```python
from build123d import *

# Parameters (mm, degrees)
F0_W     = 449.58
F0_H     = 176.784
F1_DEPTH = 70.866
F2_R     = 38.835317
F2_R_2   = 41.172166
F3_DEPTH = 25.4


with BuildPart() as f1:
    # F0 (on Top) → F1 (new body)
    with BuildSketch(Plane.XY):
        with Locations((-0.463787, -9.675345)):
            Rectangle(F0_W, F0_H)
    extrude(amount=F1_DEPTH)

    # F2 (on Front) → F3 (join)
    with BuildSketch(Plane.XZ):
        with Locations((-143.220037, 0)):
            Circle(F2_R)
        with Locations((175.135151, 0)):
            Circle(F2_R_2)
    extrude(amount=F3_DEPTH)


solid = f1.part
```
Input: part model. Units: mm. Frame: model coordinates. A direction names the side the tool comes from. Coordinates: 2 decimals unless noted, no trailing zeros. Loops run counter-clockwise (first coordinate to the right, second up) from the corner with the lowest first, then second, coordinate; pieces in that order, holes last. Notation, with made-up numbers: M 78.5,8 L 119.5,8 A15 ccw 119.5,21 Z; hole C -20,6.25 d2. An arc over 180 degrees is marked long. Use a Markdown table: item, result. Add a question column.
1) Section B-B, the plane y = -19. Return the cut outline in (x, z).
2) Set-up query: faces 1 (the flat face through (175, 0, -16)), 2 (the flat face through (-4, 78.717, 35)), 3 (the flat face through (-144, -25.4, -15)). Return all of +Z, -Z, +X, -X, +Y, -Y with unobstructed straight access to the full face (end or side cutting, diameter ignored); none if empty.
3) Section D-D, the plane y = 11. Return the cut outline in (x, z).
4) Line query: L1, parallel to Z at x = 111, y = -8; L2, parallel to Y at x = -159.5, z = -1.5. Output: solid intervals per line, ascending. Write a range as from..to.
5) Section A-A, the plane z = -13. Return the cut outline in (x, y), plus the area to 3 significant figures.
6) Section C-C, the plane x = -166.5. Return the cut outline in (y, z).
7) Pin query (flat end, axial travel): P1, Ø19.5, axis at x = -139.5, z = -13.5, coming from the -Y side; P2, Ø4, axis at x = -41.5, y = -77, coming from the -Z side; P3, Ø1.5, axis at y = -4, z = -30, coming from the +X side. Return the tip coordinate at first contact, or that it passes through.
Answer below:
| question | item | result |
|---|---|---|
| 1 | outline | M -225.25,0 L -182.06,0 A38.84 ccw -104.38,0 L 133.96,0 A41.17 ccw 216.31,0 L 224.33,0 L 224.33,70.87 L -225.25,70.87 Z |
| 2 | face 1 | -Z, +X, -X, +Y |
| 2 | face 2 | +Z, -Z, +X, -X, +Y |
| 2 | face 3 | -Z, +X, -X, -Y |
| 3 | outline | M -225.25,0 L 224.33,0 L 224.33,70.87 L -225.25,70.87 Z |
| 4 | L1 | 0..70.87 |
| 4 | L2 | -25.4..0 |
| 5 | outline | M -179.81,-25.4 L -106.63,-25.4 L -106.63,0 L -179.81,0 Z; M 136.07,-25.4 L 214.2,-25.4 L 214.2,0 L 136.07,0 Z |
| 5 | area | 3,840 mm2 |
| 6 | outline | M -98.07,0 L -25.4,0 L -25.4,-31.08 L 0,-31.08 L 0,0 L 78.72,0 L 78.72,70.87 L -98.07,70.87 Z |
| 7 | P1 | y = -25.4 |
| 7 | P2 | z = 0 |
| 7 | P3 | x = 204.11 |
